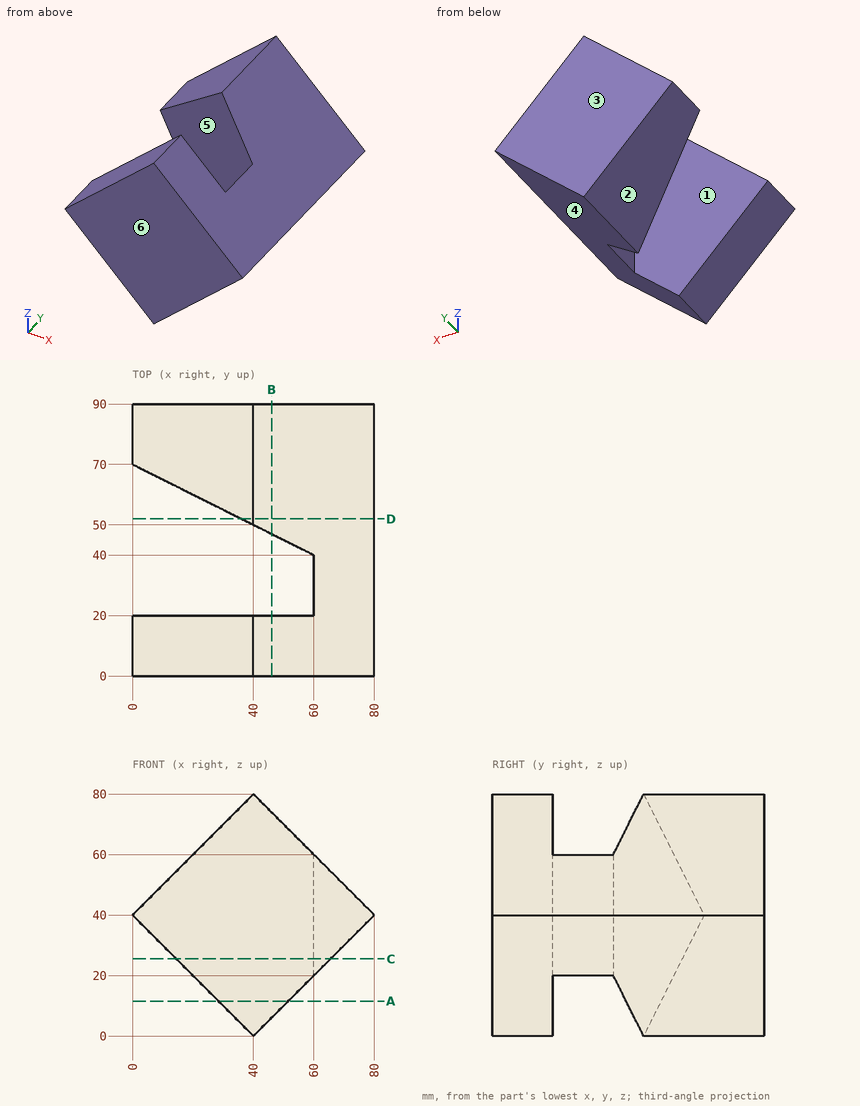
Job drawing, mm, ordinate dimensions from the low corner. One solid piece. A direction names the side the tool comes from. Round coordinates to 2 decimals unless told otherwise and drop trailing zeros. Loops run counter-clockwise (first coordinate to the right, second up) from the corner with the lowest first, then second, coordinate; pieces in that order, holes last. Notation, with made-up numbers: (10.5, 2.25) -> (36.5, 2.25) arc R16 cw to (36.5, 8.25) -> close; hole circle Ø11 at (65.25, 39). An arc over 180 degrees is marked (long way). One line per item, written item: value. Start each with the question number.
Q1. Cut at A-A on z = 11.5. List the corners of the cut face in (x, y), plus the area to 3 significant figures.
Q2. Cut at D-D on y = 52. List the corners of the cut face in (x, z), plus the area to 3 significant figures.
Q3. Two-plate mould, pull along Y, no slides. Class the marked faces 3, 4, 5 and 6: released by +Y, released by -Y, zero draft, split by the parting line, or undercut.
Q4. Probe line 1 along Y through (x, z) = (26.5, 39); line 2 along Y through (x, z) = (31, 50); line 3 along Z through (x, y) = (33.5, 65.5). List the from-to ranges inside material, lowest first.
Q5. Drop flat-ended pins along their axis: pin 1 Ø1 at (x, y) = (14.5, 65) entering from +Z; pin 2 Ø12 at (y, z) = (34.5, 21.5) entering from -X; pin 3 Ø5 at (x, y) = (51, 60) entering from -Z. Give the stop position or say it passes through.
Q6. Cut at C-C on z = 25.5. List the corners of the cut face in (x, y).
Q7. 3-axis set-ups, long thin cutter, end or side, ignore diameter. For the marked faces 1 and 2: which of +Z, -Z, +X, -X, +Y, -Y reach the whole face in a straight line?
Q8. Cut at B-B on x = 46. List the corners of the cut face in (y, z).
Computed:
1. outline: (28.5, 0) -> (51.5, 0) -> (51.5, 20) -> (28.5, 20) -> close; (28.5, 55.75) -> (51.5, 44.25) -> (51.5, 90) -> (28.5, 90) -> close
1. area: 1,380 mm²
2. outline: (36, 4) -> (40, 0) -> (80, 40) -> (40, 80) -> (36, 76) -> close
2. area: 1,900 mm²
3. face 3: released by +Y
3. face 4: zero draft
3. face 5: undercut
3. face 6: released by -Y
4. line 1: 0 to 20, 56.75 to 90
4. line 2: 0 to 20, 54.5 to 90
4. line 3: 6.5 to 73.5
5. pin 1: z = 55
5. pin 2: x = 59
5. pin 3: z = 8.5
6. outline: (14.5, 0) -> (65.5, 0) -> (65.5, 90) -> (14.5, 90) -> (14.5, 62.75) -> (60, 40) -> (60, 20) -> (14.5, 20) -> close
7. face 1: +Z, -Z, -X
7. face 2: -Z, -X, +Y, -Y
8. outline: (0, 6) -> (20, 6) -> (20, 74) -> (0, 74) -> close; (47, 6) -> (90, 6) -> (90, 74) -> (47, 74) -> close
